Could you check a few things on this model? Use its own coordinates, in mm. A direction names the side the tool comes from. Give positions to 0.01 mm unless a question says otherwise; leave off trailing zeros. Order: outer loops, then holes, each group sorted by start corner. A loop starts at its lowest first (then second) coordinate and runs counter-clockwise, first axis right, second up. Notation, with made-up numbers: M 65.5,57 L 122.5,57 A17 ccw 122.5,89 Z; hole C 23.5,11.25 d1. An arc over 180 degrees is marked long. Answer in a Markdown table with one row per item. Add a question column.
```python
from build123d import *

# Parameters (mm, degrees)
BOSS_EXTRUDE1_DEPTH = 3.175
SKETCH2_R           = 1.5875
CUT_EXTRUDE1_DEPTH  = 4.175


with BuildPart() as part:
    # Sketch1 → Boss-Extrude1 (new body)
    with BuildSketch(Plane(origin=(0, 0, 0), x_dir=(1, 0, 0), z_dir=(0, 1, 0))):
        Polygon((0, 50.8), (0, 0), (88.9, 0), (88.9, 38.1), (38.1, 38.1), (38.1, 50.8), align=None)
    extrude(amount=BOSS_EXTRUDE1_DEPTH)

    # Sketch2 → Cut-Extrude1 (cut, through all)
    with BuildSketch(Plane(origin=(0, 3.175, 0), x_dir=(1, 0, 0), z_dir=(0, 1, 0))):
        with Locations((6.35, 44.45)):
            Circle(SKETCH2_R)
        with Locations((31.75, 44.45)):
            Circle(SKETCH2_R)
        with Locations((31.75, 31.75)):
            Circle(SKETCH2_R)
        with Locations((6.35, 31.75)):
            Circle(SKETCH2_R)
        with Locations((6.35, 6.35)):
            Circle(SKETCH2_R)
        with Locations((31.75, 6.35)):
            Circle(SKETCH2_R)
        with Locations((82.55, 6.35)):
            Circle(SKETCH2_R)
        with Locations((82.55, 31.75)):
            Circle(SKETCH2_R)
        with Locations((57.15, 31.75)):
            Circle(SKETCH2_R)
        with Locations((57.15, 6.35)):
            Circle(SKETCH2_R)
        with Locations((44.45, 6.35)):
            Circle(SKETCH2_R)
        with Locations((44.45, 31.75)):
            Circle(SKETCH2_R)
    extrude(amount=-CUT_EXTRUDE1_DEPTH, mode=Mode.SUBTRACT)


solid = part.part
```
1. Suppose I cut it at B-B on z = -31.75. List the corners of the cut face in (x, y) for me (1 decimal).
2. Thinking about a two-plate mould opening in X: for faces 1 (the flat face through (88.9, 2, -19)), 2 (the cylindrical face through (32.48, 1.61, -43.04)), 3 (the flat face through (44, 2, 0)), which applies, pulls with the +X half, pulls with the -X half, needs draft (parallel to the pull), parting line crosses it, or undercut?
3. Will these pins go through, and if not, where does the flat tip stop? P1, Ø4, axis at x = 31.75, z = -44.45, coming from the -Y side; P2, Ø1.6, axis at y = 2.5, z = -45.5, coming from the +X side.
4. Suppose I cut it at D-D on z = -44.45. List the corners of the cut face in (x, y) for me (1 decimal), plus the area to 3 significant figures.
5. If I drill on line 1 along Z through (x, y) = (6.35, 1.3); line 2 along X through (y, z) = (1.45, -31.75); line 3 along Z through (x, y) = (82.55, 1.9), over which ranges is the centre line in solid material (lowest first)? Write a range as [from, to].
6. For faces 4 (the cylindrical face through (84, 1.6, -5.7)), 5 (the flat face through (38.1, 2, -44)), which set-ups out of +Z, -Z, +X, -X, +Y, -Y let a thin tool reach every point of the face, with its end or its side?
7. Suppose I cut it at C-C on x = 82.55. List the corners of the cut face in (y, z) for me (1 decimal), plus the area to 3 significant figures.
8. Suppose I cut it at A-A on x = 31.75. List the corners of the cut face in (y, z) for me (1 decimal).
Findings below:
| question | item | result |
|---|---|---|
| 1 | outline | M 0,0 L 4.8,0 L 4.8,3.2 L 0,3.2 Z; M 7.9,0 L 30.2,0 L 30.2,3.2 L 7.9,3.2 Z; M 33.3,0 L 42.9,0 L 42.9,3.2 L 33.3,3.2 Z; M 46,0 L 55.6,0 L 55.6,3.2 L 46,3.2 Z; M 58.7,0 L 81,0 L 81,3.2 L 58.7,3.2 Z; M 84.1,0 L 88.9,0 L 88.9,3.2 L 84.1,3.2 Z |
| 2 | face 1 | pulls with the +X half |
| 2 | face 2 | undercut |
| 2 | face 3 | needs draft |
| 3 | P1 | y = 0 |
| 3 | P2 | x = 38.1 |
| 4 | outline | M 0,0 L 4.8,0 L 4.8,3.2 L 0,3.2 Z; M 7.9,0 L 30.2,0 L 30.2,3.2 L 7.9,3.2 Z; M 33.3,0 L 38.1,0 L 38.1,3.2 L 33.3,3.2 Z |
| 4 | area | 101 mm2 |
| 5 | line 1 | [-50.8, -46.04], [-42.86, -33.34], [-30.16, -7.94], [-4.76, 0] |
| 5 | line 2 | [0, 4.76], [7.94, 30.16], [33.34, 42.86], [46.04, 55.56], [58.74, 80.96], [84.14, 88.9] |
| 5 | line 3 | [-38.1, -33.34], [-30.16, -7.94], [-4.76, 0] |
| 6 | face 4 | +Y, -Y |
| 6 | face 5 | -Z, +X, +Y, -Y |
| 7 | outline | M 0,-38.1 L 3.2,-38.1 L 3.2,-33.3 L 0,-33.3 Z; M 0,-30.2 L 3.2,-30.2 L 3.2,-7.9 L 0,-7.9 Z; M 0,-4.8 L 3.2,-4.8 L 3.2,0 L 0,0 Z |
| 7 | area | 101 mm2 |
| 8 | outline | M 0,-50.8 L 3.2,-50.8 L 3.2,-46 L 0,-46 Z; M 0,-42.9 L 3.2,-42.9 L 3.2,-33.3 L 0,-33.3 Z; M 0,-30.2 L 3.2,-30.2 L 3.2,-7.9 L 0,-7.9 Z; M 0,-4.8 L 3.2,-4.8 L 3.2,0 L 0,0 Z |
